Geometry check sheet. Reference: the model listing, model coordinates, mm. Give positions to 0.01 mm unless a question says otherwise; leave off trailing zeros. Loops run counter-clockwise (first coordinate to the right, second up) from the corner with the lowest first, then second, coordinate; pieces in that order, holes last. Notation, with made-up numbers: (-13, -35.5) -> (-8, -35.5) arc R23 ccw to (-8, -25.5) -> close; hole circle Ø3 at (88.5, 77). An arc over 180 degrees is marked (long way). Answer as a JSON object with one key per item and string values.
from build123d import *

# Parameters (mm, degrees)
F0_W     = 254
F0_H     = 152.4
F1_DEPTH = 914.4
F3_D     = 76.2
F4_R     = 126.99999


# Not quite as in the source:
# - a fillet or chamfer is up to 0.001 mm smaller than in the source, because OpenCascade refuses the exact size


with BuildPart() as f1:
    # F0 (on Front) → F1 (new body, symmetric)
    with BuildSketch(Plane.XZ):
        Rectangle(F0_W, F0_H)
    extrude(amount=F1_DEPTH, both=True)

    # F3 (through all)
    with Locations(Plane.XY.offset(76.2)):
        with Locations((0, 762), (0, -762)):
            Hole(F3_D / 2)

    # F4 (radius 127 in the source; OpenCascade refuses exactly that, so slightly less here)
    f4_edges = [f1.edges().sort_by_distance(p)[0] for p in [
        (127, -914.4, 0),
        (-127, -914.4, 0),
        (127, 914.4, 0),
        (-127, 914.4, 0),
    ]]
    fillet(f4_edges, radius=F4_R)


solid = f1.part
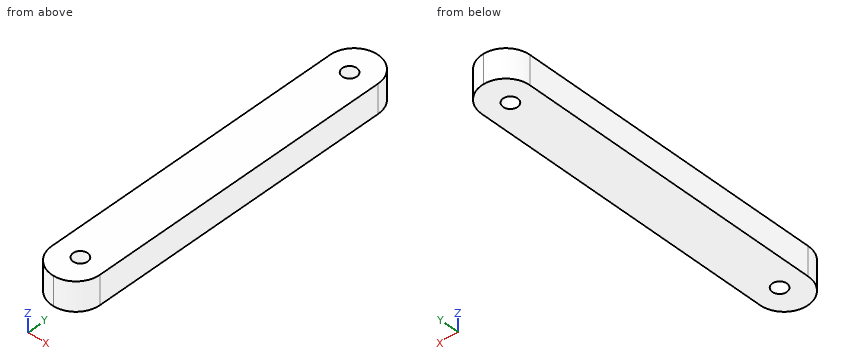
1) Material ranges on line 1 along Y through (x, z) = (-5, 21); line 2 along Y through (x, z) = (-27, 38); line 3 along Y through (x, z) = (-59.5, 54), recorded low to high. Write a range as from..to.
Geometry check:
{"line 1": "y = -914.3..-799.77, -724.23..724.23, 799.77..914.3", "line 2": "y = -911.5..-788.88, -735.12..735.12, 788.88..911.5", "line 3": "y = -899.6..899.6"}
2) Section check C-C on x = -86.5. Record the cut outline in (y, z), plus the area to 3 significant figures.
Geometry check:
{"outline": "(-880.39, -76.2) -> (880.39, -76.2) -> (880.39, 76.2) -> (-880.39, 76.2) -> close", "area": "268,000 mm2"}
3) Section check B-B on z = -59. Count the separate pieces of the cut face and the enclosed holes in it, plus the area to 3 significant figures.
Geometry check:
{"separate pieces": "1", "enclosed holes": "2", "area": "442,000 mm2"}
4) Section check A-A on y = -762. Record the cut outline in (x, z), plus the area to 3 significant figures.
Geometry check:
{"outline": "(-127, -76.2) -> (-38.1, -76.2) -> (-38.1, 76.2) -> (-127, 76.2) -> close; (38.1, -76.2) -> (127, -76.2) -> (127, 76.2) -> (38.1, 76.2) -> close", "area": "27,100 mm2"}
5) Depth check by flat-ended pin: P1, Ø2, axis at x = 14.5, z = 60.5, coming from the -Y side; P2, Ø12, axis at x = 21, z = -39.5, coming from the -Y side; P3, Ø5, axis at x = 56.5, z = 14, coming from the -Y side. Enter the tip coordinate at first touch or a pass-through.
Geometry check:
{"P1": "stops at y = -913.68", "P2": "stops at y = -913.51", "P3": "stops at y = -902.35"}
6) Section check D-D on x = 81. Record the cut outline in (y, z).
Geometry check:
{"outline": "(-885.22, -76.2) -> (885.22, -76.2) -> (885.22, 76.2) -> (-885.22, 76.2) -> close"}
